Could you check a few things on this model? Use its own coordinates, in mm. A direction names the side the tool comes from. Give positions to 0.01 mm unless a question says otherwise; leave off trailing zeros. Loops run counter-clockwise (first coordinate to the right, second up) from the corner with the lowest first, then second, coordinate; pieces in that order, holes last. Notation, with made-up numbers: (27.5, -18) - (54.5, -18) arc R28 ccw to (54.5, 9) - close; hole circle Ø9 at (-6, 50). An arc over 180 degrees is marked (long way). Write each question's results on one line, items separated by ' | '. Start each with the question number.
1) I'm going to push flat-ended pins straight in: pin 1 (3 mm diameter, centred on x = 15.5, z = -14.5, fed in from -Y); pin 2 (12.5 mm diameter, centred on x = 18, y = -12, fed in from -Z); pin 3 (4.5 mm diameter, centred on x = 2.5, z = -25, fed in from -Y). Where does each tip first touch, or does it pass through?
2) I want a section at B-B, the plane x = 16.25. Write out the boundary of the cut face in (y, z).
3) On a 3-axis mill with a long thin cutter (end or side, diameter ignored), from which of +Z, -Z, +X, -X, +Y, -Y can I reach the whole of each face in a straight line? I mean faces 1 (the face through (2, -15, -22)), 2 (the face through (30, -10, -4)), 3 (the face through (17, -5, -18)). Say none if no direction works.
4) If I drill on probe 1 along Y at (x, z) = (16, -21.5); probe 2 along X at (y, z) = (-14.5, -13.25), over which ranges is the centre line in solid material (lowest first)? Write a range as [from, to].
5) I want a section at A-A, the plane z = -18. Write out the boundary of the cut face in (x, y), and give its area (3 significant figures).
from build123d import *

# Parameters (mm, degrees)
F1_DEPTH     = 30
F3_DEPTH     = 26
F4_R         = 2
F5_T1_DEPTH  = 4
F5_T3_DEPTH  = 14
F5_T5_DEPTH  = 8
F5_T7_DEPTH  = 8
F5_S11_W     = 2
F5_S11_H     = 2
F5_T12_DEPTH = 2
F5_S17_W     = 2
F5_S17_H     = 2
F5_T18_DEPTH = 2


# Not quite as in the source:
# - a fillet or chamfer that OpenCascade refuses, or shapes differently, is made with other operations: its cross-section is extruded or revolved along the edge and cut away or added


with BuildPart() as f1:
    # F0 (on Right) → F1 (new body)
    with BuildSketch(Plane.YZ):
        Polygon((0, -30), (0, 0), (-30, 0), (-30, -15), (-15, -15), (-15, -30), align=None)
    extrude(amount=F1_DEPTH)

    # F2 (on face) → F3 (cut)
    with BuildSketch(Plane.YZ.offset(30)):
        Polygon((-30, -5), (-30, -15), (-15, -15), (-15, -30), (-5, -30), (-5, -5), align=None)
    extrude(amount=-F3_DEPTH, mode=Mode.SUBTRACT)

    # F4
    f4_edges = [f1.edges().sort_by_distance(p)[0] for p in [
        (15, -30, 0),
        (15, 0, 0),
        (0, -15, 0),
        (0, 0, -15),
        (15, 0, -30),
        (30, 0, -15),
        (30, -15, 0),
    ]]
    fillet(f4_edges, radius=F4_R)

    # F5: fillet of radius 2 on 5 edges, made by hand

    # F5_s2 → F5_t1 (join)
    with BuildSketch(Plane.YZ):
        with BuildLine():
            ThreePointArc((-17, -15), (-15.5857864376, -15.5857864376), (-15, -17))
            Line((-15, -17), (-15, -15))
            Line((-15, -15), (-17, -15))
        make_face()
    extrude(amount=F5_T1_DEPTH)

    # F5_s4 → F5_t3 (cut)
    with BuildSketch(Plane.YZ.offset(-5)):
        with BuildLine():
            ThreePointArc((-13, -30), (-14.4142135624, -29.4142135624), (-15, -28))
            Line((-15, -28), (-15, -30))
            Line((-15, -30), (-13, -30))
        make_face()
        with BuildLine():
            ThreePointArc((-30, -13), (-29.4142135624, -14.4142135624), (-28, -15))
            Line((-28, -15), (-30, -15))
            Line((-30, -15), (-30, -13))
        make_face()
    extrude(amount=F5_T3_DEPTH, mode=Mode.SUBTRACT)

    # F5_s6 → F5_t5 (cut)
    with BuildSketch(Plane.XZ.offset(2)):
        with BuildLine():
            ThreePointArc((30, -28), (29.4142135624, -29.4142135624), (28, -30))
            Line((28, -30), (30, -30))
            Line((30, -30), (30, -28))
        make_face()
    extrude(amount=F5_T5_DEPTH, mode=Mode.SUBTRACT)

    # F5_s8 → F5_t7 (cut)
    with BuildSketch(Plane.XY.offset(-10)):
        with BuildLine():
            ThreePointArc((30, -28), (29.4142135624, -29.4142135624), (28, -30))
            Line((28, -30), (30, -30))
            Line((30, -30), (30, -28))
        make_face()
    extrude(amount=F5_T7_DEPTH, mode=Mode.SUBTRACT)


with BuildPart() as f5_tool10:
    # F5_s11 → F5_t12 (new body)
    with BuildSketch(Plane.YZ.offset(28)):
        with Locations((-29, -1)):
            Rectangle(F5_S11_W, F5_S11_H)
    extrude(amount=F5_T12_DEPTH)

    # F5_s13 → F5_t14 (revolve, cut)
    with BuildSketch(Plane(origin=(28, -28, -2), x_dir=(0, 0.7071067812, -0.7071067812), z_dir=(0, -0.7071067812, -0.7071067812))):
        with BuildLine():
            ThreePointArc((0, -2), (2, 0), (0, 2))
            Line((0, 2), (0, -2))
        make_face()
    revolve(axis=Axis((28, -28, -2), (1, 0, 0)), mode=Mode.SUBTRACT)


with BuildPart() as f1_1:
    add(f1.part)

    # F5_t9: cut F5_tool10
    add(f5_tool10.part, mode=Mode.SUBTRACT)


with BuildPart() as f5_tool16:
    # F5_s17 → F5_t18 (new body)
    with BuildSketch(Plane.YZ.offset(28)):
        with Locations((-1, -29)):
            Rectangle(F5_S17_W, F5_S17_H)
    extrude(amount=F5_T18_DEPTH)

    # F5_s19 → F5_t20 (revolve, cut)
    with BuildSketch(Plane(origin=(28, -2, -28), x_dir=(0, -0.7071067812, 0.7071067812), z_dir=(0, 0.7071067812, 0.7071067812))):
        with BuildLine():
            ThreePointArc((0, -2), (2, 0), (0, 2))
            Line((0, 2), (0, -2))
        make_face()
    revolve(axis=Axis((28, -2, -28), (1, 0, 0)), mode=Mode.SUBTRACT)


with BuildPart() as f1_2:
    add(f1_1.part)

    # F5_t15: cut F5_tool16
    add(f5_tool16.part, mode=Mode.SUBTRACT)


solid = f1_2.part
Answers:
1) pin 1: stops at y = -5 | pin 2: stops at z = -5 | pin 3: stops at y = -15
2) outline: (-30, -5) - (-5, -5) - (-5, -30) - (-2, -30) arc R2 ccw to (0, -28) - (0, -2) arc R2 ccw to (-2, 0) - (-28, 0) arc R2 ccw to (-30, -2) - close
3) face 1: -Z, +X, -X, -Y | face 2: +Z, -Z, +X, +Y, -Y | face 3: -Z, +X, -Y
4) probe 1: y = [-5, 0] | probe 2: x = [0, 4]
5) outline: (0, -15) - (4, -15) - (4, -5) - (30, -5) - (30, -2) arc R2 ccw to (28, 0) - (2, 0) arc R2 ccw to (0, -2) - close | area: 188 mm2
